The listing builds one solid part. Answer for the finished solid, in the listing's coordinates (mm). Face numbers are marked on the shaded views. Round coordinates to 2 decimals unless told otherwise and drop trailing zeros. Loops run counter-clockwise (first coordinate to the right, second up) from the corner with the lowest first, then second, coordinate; pieces in that order, holes last. Notation, with made-up numbers: (-17, 23.5) -> (8, 23.5) arc R23 cw to (8, 40.5) -> close; hole circle Ø4 at (-2, 42). An arc over 180 degrees is marked (long way). Use a Markdown table: item, result. Add a question column.
Q1. Section C-C on y = -8 is taken. Give the vertices of the cut face in (x, z), then the cut area to 3 significant figures.
Q2. Section B-B on x = 0.5 is taken. Give the vertices of the cut face in (y, z), then the cut area to 3 significant figures.
Q3. For a pull along X with two mould halves and no side action, classify the marked faces 1, 2 and 3 as released by +X, released by -X, zero draft, split by the parting line, or undercut.
Q4. Section A-A on z = -2.5 is taken. Give the number of separate pieces and of enclosed holes in the cut face, then the cut area to 3 significant figures.
Q5. Given pin 1 Ø1 at (x, z) = (3, -2.5) entering from -Y, flat-ended and moving along its own axis, determine where the tip first touches the part or whether it passes through.
Q6. Consider line 1 (Z direction, x = 3.5, y = 0.25). Determine where the line is inside the solid, lowest interval first.
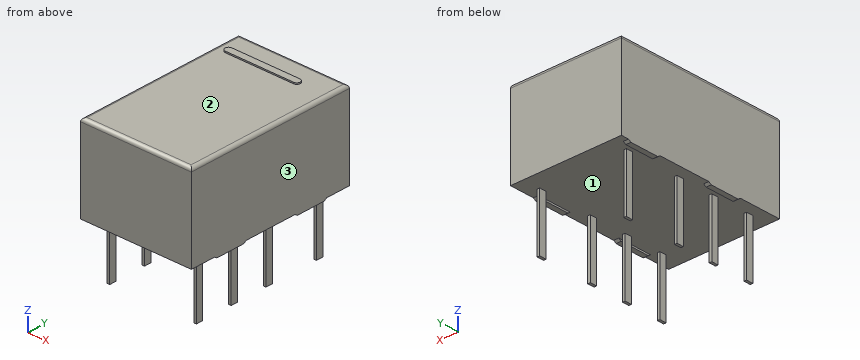
from build123d import *

# Parameters (mm, degrees)
PAD003_DEPTH = 0.3
PAD001_DEPTH = 0.18
SKETCH002_W  = 0.4
SKETCH002_H  = 0.15
PAD002_DEPTH = 3.5
SKETCH_W     = 10
SKETCH_H     = 6.5
PAD_DEPTH    = 5
POCKET_DEPTH = 0.5
FILLET_R     = 0.2
PAD004_DEPTH = 0.3


with BuildPart() as pad003:
    # Sketch005 → Pad003 (new body)
    with BuildSketch(Plane(origin=(-0.71, 1, 0), x_dir=(0, 1, 0), z_dir=(1, 0, 0))):
        Polygon((-7.33, 0.1), (-7.18, 0), (-5.48, 0), (-5.33, 0.1), align=None)
        Polygon((-2.25, 0.1), (-2.1, 0), (-0.4, 0), (-0.25, 0.1), align=None)
    extrude(amount=PAD003_DEPTH)


with BuildPart() as pad001:
    # Sketch001 → Pad001 (new body)
    with BuildSketch(Plane(origin=(0, 0, 5), x_dir=(0, -1, 0), z_dir=(0, 0, 1))):
        with BuildLine():
            Line((0.4, 0), (0.4, 4))
            ThreePointArc((0.4, 4), (0.2, 4.2), (0, 4))
            Line((0, 4), (0, 0))
            ThreePointArc((0, 0), (0.2, -0.2), (0.4, 0))
        make_face()
    extrude(amount=PAD001_DEPTH)


with BuildPart() as pad002:
    # Sketch002 → Pad002 (new body)
    with BuildSketch(Plane(origin=(0, 0, 0.25), x_dir=(0, -1, 0), z_dir=(0, 0, 1))):
        Rectangle(SKETCH002_W, SKETCH002_H)
        with Locations((3.2, 0)):
            Rectangle(SKETCH002_W, SKETCH002_H)
        with Locations((5.4, 0)):
            Rectangle(SKETCH002_W, SKETCH002_H)
        with Locations((7.6, 0)):
            Rectangle(SKETCH002_W, SKETCH002_H)
        with Locations((0, 5.08)):
            Rectangle(SKETCH002_W, SKETCH002_H)
        with Locations((3.2, 5.08)):
            Rectangle(SKETCH002_W, SKETCH002_H)
        with Locations((5.4, 5.08)):
            Rectangle(SKETCH002_W, SKETCH002_H)
        with Locations((7.6, 5.08)):
            Rectangle(SKETCH002_W, SKETCH002_H)
    extrude(amount=-PAD002_DEPTH)


with BuildPart() as fillet_body:
    # Sketch → Pad (new body)
    with BuildSketch(Plane(origin=(0, 0, 0.1), x_dir=(0, -1, 0), z_dir=(0, 0, 1))):
        with Locations((3.8, 2.54)):
            Rectangle(SKETCH_W, SKETCH_H)
    extrude(amount=PAD_DEPTH)

    # Sketch003 → Pocket (cut)
    with BuildSketch(Plane(origin=(0, 0, 5.1), x_dir=(0, -1, 0), z_dir=(0, 0, 1))):
        with BuildLine():
            ThreePointArc((-0.318267, 7.6), (0.223846, 7.813173), (0.45, 8.35))
            Line((0.45, 8.35), (-2.05, 8.35))
            Line((-2.05, 8.35), (-2.05, 7.6))
            Line((-2.05, 7.6), (-0.318267, 7.6))
        make_face()
        with BuildLine():
            Line((9.6, -0.75), (12.1, -0.75))
            Line((12.1, -0.75), (12.1, 0))
            Line((10.285847, 0), (12.1, 0))
            ThreePointArc((10.285847, 0), (9.797313, -0.241845), (9.6, -0.75))
        make_face()
    extrude(amount=-POCKET_DEPTH, mode=Mode.SUBTRACT)

    # Fillet
    fillet_edges = [fillet_body.edges().sort_by_distance(p)[0] for p in [
        (-0.71, -3.8, 5.1),
        (2.54, -8.8, 5.1),
        (5.79, -3.8, 5.1),
        (2.54, 1.2, 5.1),
    ]]
    fillet(fillet_edges, radius=FILLET_R)


with BuildPart() as obj1:
    # Sketch006 → Pad004 (new body)
    with BuildSketch(Plane.YZ.offset(5.79)):
        Polygon((-7.33, 0.1), (-7.18, 0), (-5.48, 0), (-5.33, 0.1), align=None)
        Polygon((-2.25, 0.1), (-2.1, 0), (-0.4, 0), (-0.25, 0.1), align=None)
    extrude(amount=-PAD004_DEPTH)

    add(pad003.part)
    add(pad001.part)
    add(pad002.part)
    add(fillet_body.part)


solid = obj1.part
Checked values:
| question | item | result |
|---|---|---|
| 1 | outline | (-0.71, 0.1) -> (5.79, 0.1) -> (5.79, 4.9) arc R0.2 ccw to (5.59, 5.1) -> (-0.51, 5.1) arc R0.2 ccw to (-0.71, 4.9) -> close |
| 1 | area | 32.5 mm2 |
| 2 | outline | (-8.8, 0.1) -> (1.2, 0.1) -> (1.2, 4.9) arc R0.2 ccw to (1, 5.1) -> (0, 5.1) -> (0, 5.18) -> (-0.4, 5.18) -> (-0.4, 5.1) -> (-8.6, 5.1) arc R0.2 ccw to (-8.8, 4.9) -> close |
| 2 | area | 50.0 mm2 |
| 3 | face 1 | undercut |
| 3 | face 2 | zero draft |
| 3 | face 3 | released by +X |
| 4 | separate pieces | 8 |
| 4 | enclosed holes | 0 |
| 4 | area | 0.480 mm2 |
| 5 | pin 1 | passes through |
| 6 | line 1 | z = 0.1 to 5.1 |
